Part print with two shaded views. Sizes in mm from the minimum x, y, z corner. A direction names the side the tool comes from. Give positions to 0.01 mm unless a question says otherwise; leave off trailing zeros. Write each loop counter-clockwise with the first axis right and the second up, starting at its lowest first coordinate (ties: lowest second). Pieces come first, ordered by that corner, then holes. Notation, with made-up numbers: (67, 43) - (97, 43) arc R25 cw to (97, 66) - close; hole circle Ø5 at (-10.5, -21.5). An arc over 180 degrees is marked (long way). Answer as a JSON object with one key per item and string values. Group by question number.
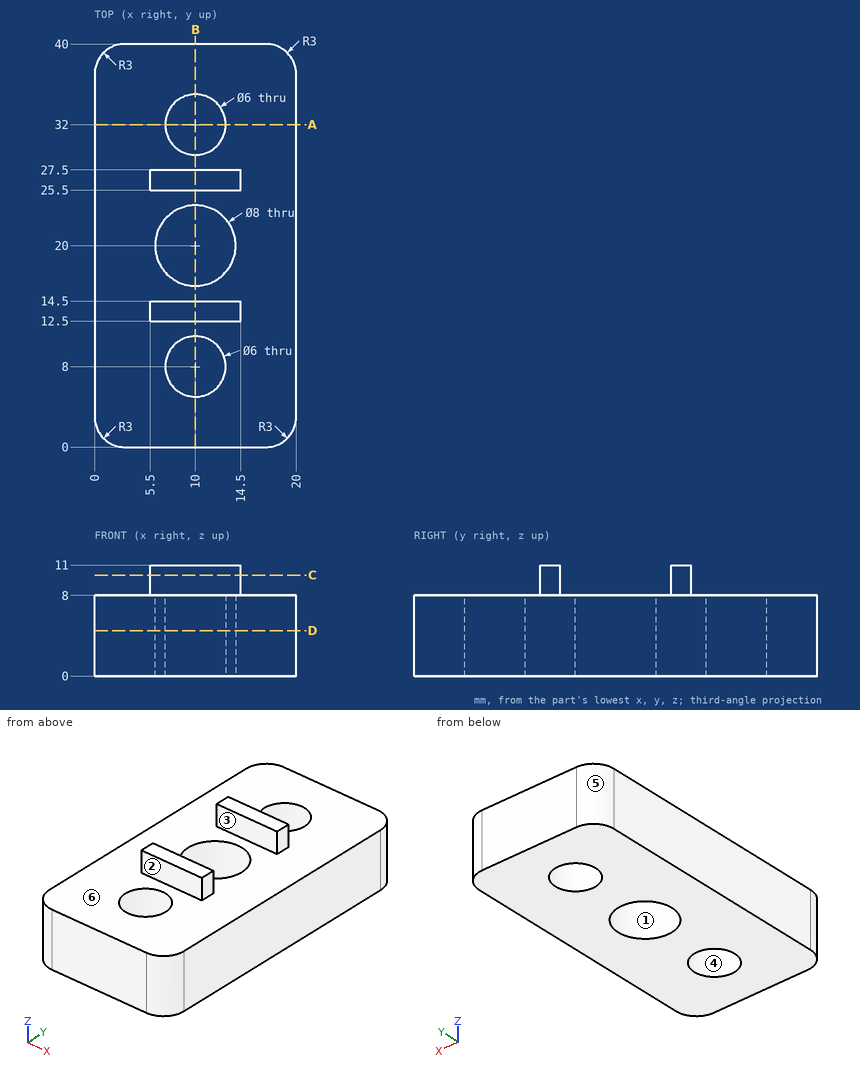
1) Which spindle directions (+Z, -Z, +X, -X, +Y, -Y) get a long thin tool onto all of the face, cutting with end or side? Do the marked faces 1, 2 and 3. Say none if no direction does.
2) Saw through at C-C (z = 10). List the corners of the cut face in (x, y), and give its area (3 significant figures).
3) Saw through at A-A (y = 32). List the corners of the cut face in (x, z).
4) Saw through at B-B (x = 10). List the corners of the cut face in (y, z).
5) Drill centre lines: line 1 along Y through (x, z) = (10, 4.75); line 2 along Y through (x, z) = (7.75, 7.25); line 3 along Y through (x, z) = (9.5, 9.5). Where is each one in solid material? Low to high. Write a range as from..to.
6) Two-plate mould, pull along X, no slides. Class the marked faces 4, 5 and 6: +X half, -X half, draft (parallel to the pull), parting line (faces both ways), or undercut.
7) Drop flat-ended pins along their axis: P1, Ø1.6, axis at y = 26.5, z = 10, coming from the -X side; P2, Ø1, axis at y = 27, z = 10, coming from the +X side; P3, Ø1.5, axis at x = 11, z = 10, coming from the +Y side. Give the stop position or say it passes through.
8) Saw through at D-D (z = 4.5). List the corners of the cut face in (x, y), and give its area (3 significant figures).
Checks:
{
 "1": {"face 1": "+Z, -Z", "face 2": "+Z, +X, -X, -Y", "face 3": "+Z, +X, -X"},
 "2": {"outline": "(5.5, 12.5) - (14.5, 12.5) - (14.5, 14.5) - (5.5, 14.5) - close; (5.5, 25.5) - (14.5, 25.5) - (14.5, 27.5) - (5.5, 27.5) - close", "area": "36.0 mm2"},
 "3": {"outline": "(0, 0) - (7, 0) - (7, 8) - (0, 8) - close; (13, 0) - (20, 0) - (20, 8) - (13, 8) - close"},
 "4": {"outline": "(0, 0) - (5, 0) - (5, 8) - (0, 8) - close; (11, 0) - (16, 0) - (16, 8) - (14.5, 8) - (14.5, 11) - (12.5, 11) - (12.5, 8) - (11, 8) - close; (24, 0) - (29, 0) - (29, 8) - (27.5, 8) - (27.5, 11) - (25.5, 11) - (25.5, 8) - (24, 8) - close; (35, 0) - (40, 0) - (40, 8) - (35, 8) - close"},
 "5": {"line 1": "0..5, 11..16, 24..29, 35..40", "line 2": "0..6.02, 9.98..16.69, 23.31..30.02, 33.98..40", "line 3": "12.5..14.5, 25.5..27.5"},
 "6": {"face 4": "undercut", "face 5": "-X half", "face 6": "draft"},
 "7": {"P1": "x = 5.5", "P2": "x = 14.5", "P3": "y = 27.5"},
 "8": {"outline": "(0, 3) arc R3 ccw to (3, 0) - (17, 0) arc R3 ccw to (20, 3) - (20, 37) arc R3 ccw to (17, 40) - (3, 40) arc R3 ccw to (0, 37) - close; hole circle Ø8 at (10, 20); hole circle Ø6 at (10, 8); hole circle Ø6 at (10, 32)", "area": "685 mm2"}
}
